Part print with two shaded views. Sizes in mm from the minimum x, y, z corner. A direction names the side the tool comes from. Coordinates: 2 decimals unless noted, no trailing zeros. Loops run counter-clockwise (first coordinate to the right, second up) from the corner with the lowest first, then second, coordinate; pieces in that order, holes last. Notation, with made-up numbers: (42, 66) -> (95, 66) arc R30 cw to (95, 99) -> close; hole circle Ø11 at (-13, 58). An arc over 180 degrees is marked (long way). One line per item, written item: value. Start each with the question number.
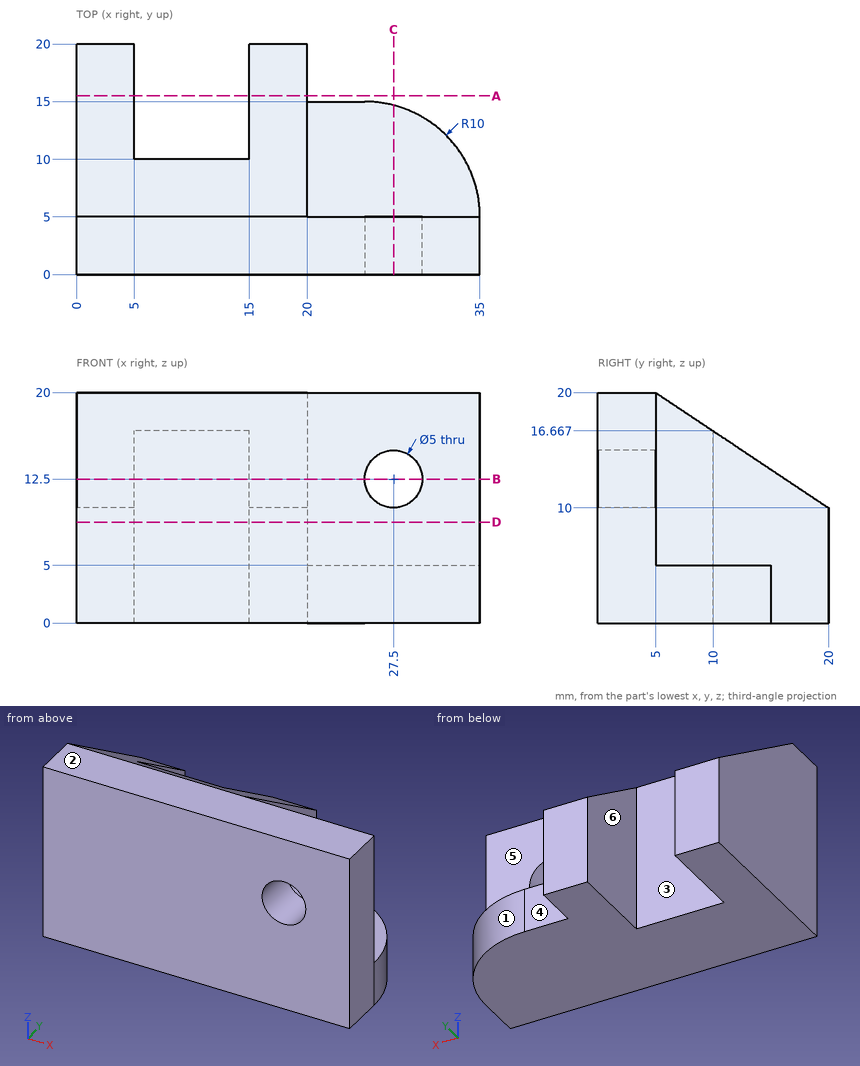
Item 1: Band-saw the part on D-D, the plane z = 8.75. List the corners of the cut face in (x, y), and give its area (3 significant figures).
Item 2: Band-saw the part on A-A, the plane y = 15.5. List the corners of the cut face in (x, z), and give its area (3 significant figures).
Item 3: Two-plate mould, pull along X, no slides. Class the marked faces 1, 2 and 3: +X half, -X half, draft (parallel to the pull), parting line (faces both ways), or undercut.
Item 4: Band-saw the part on B-B, the plane z = 12.5. List the corners of the cut face in (x, y).
Item 5: Band-saw the part on C-C, the plane x = 27.5. List the corners of the cut face in (y, z).
Item 6: Drop flat-ended pins along their axis: pin 1 Ø4 at (y, z) = (13.5, 15) entering from +X; pin 2 Ø5 at (y, z) = (16, 6) entering from +X (1 decimal); pin 3 Ø5 at (x, y) = (24.5, 10) entering from +Z. Give the stop position or say it passes through.
Item 7: Tool access for the marked faces 4, 5 and 6: list every direction of +Z, -Z, +X, -X, +Y, -Y with a clear straight run to the whole face (end or side of a thin tool).
Item 8: Probe probe 1 along X at (y, z) = (1.1, 12.5); probe 2 along Z at (x, y) = (27.5, 3.65); probe 3 along X at (y, z) = (16.5, 3). List the from-to ranges inside material, lowest first.
Worked out:
1. outline: (0, 0) -> (35, 0) -> (35, 5) -> (20, 5) -> (20, 20) -> (15, 20) -> (15, 10) -> (5, 10) -> (5, 20) -> (0, 20) -> close
1. area: 375 mm²
2. outline: (0, 0) -> (5, 0) -> (5, 13) -> (0, 13) -> close; (15, 0) -> (20, 0) -> (20, 13) -> (15, 13) -> close
2. area: 130 mm²
3. face 1: +X half
3. face 2: draft
3. face 3: undercut
4. outline: (0, 0) -> (25, 0) -> (25, 5) -> (20, 5) -> (20, 16.25) -> (15, 16.25) -> (15, 10) -> (5, 10) -> (5, 16.25) -> (0, 16.25) -> close; (30, 0) -> (35, 0) -> (35, 5) -> (30, 5) -> close
5. outline: (0, 0) -> (14.68, 0) -> (14.68, 5) -> (5, 5) -> (5, 10) -> (0, 10) -> close; (0, 15) -> (5, 15) -> (5, 20) -> (0, 20) -> close
6. pin 1: stops at x = 20
6. pin 2: stops at x = 29.9
6. pin 3: stops at z = 5
7. face 4: +Z, -Z, +X, +Y
7. face 5: +Z, +X, +Y
7. face 6: +Z, -Z, +Y
8. probe 1: x = 0 to 25, 30 to 35
8. probe 2: z = 0 to 10, 15 to 20
8. probe 3: x = 0 to 5, 15 to 20
